from build123d import *

# Parameters (mm, degrees)
SKETCH1_R           = 48.846646741
SKETCH1_R_2         = 45.593095846
BOSS_EXTRUDE1_DEPTH = 10
SKETCH2_W           = 14.682281382
SKETCH2_H           = 11.549997154
SKETCH2_W_2         = 10
SKETCH2_H_2         = 8
BOSS_EXTRUDE2_DEPTH = 15
FILLET1_R           = 4


with BuildPart() as part:
    # Sketch1 → Boss-Extrude1 (new, symmetric)
    with BuildSketch(Plane.XY):
        Circle(SKETCH1_R)
        Circle(SKETCH1_R_2, mode=Mode.SUBTRACT)
    extrude(amount=BOSS_EXTRUDE1_DEPTH, both=True)

    # Sketch2 → Boss-Extrude2 (add)
    with BuildSketch(Plane.XY.offset(10)):
        with Locations((0, 53.899768405)):
            Rectangle(SKETCH2_W, SKETCH2_H)
        with Locations((0, 53.899768405)):
            Rectangle(SKETCH2_W_2, SKETCH2_H_2, mode=Mode.SUBTRACT)
    extrude(amount=-BOSS_EXTRUDE2_DEPTH)

    # Fillet1
    fillet1_edges = [part.edges().sort_by_distance(p)[0] for p in [
        (7.341140691, 59.674766982, 2.5),
        (-7.341140691, 59.674766982, 2.5),
    ]]
    fillet(fillet1_edges, radius=FILLET1_R)


solid = part.part
Can you work these out from the model? Positions are in its coordinate system, mm. A direction names the side the tool comes from. Round coordinates to 2 decimals unless told otherwise and drop trailing zeros. Loops run counter-clockwise (first coordinate to the right, second up) from the corner with the lowest first, then second, coordinate; pieces in that order, holes last. Notation, with made-up numbers: (73, 4) - (84, 4) arc R26 ccw to (84, 38) - close; hole circle Ø1 at (72.5, 36.5). An arc over 180 degrees is marked (long way). Use CSV: the item, a comma, the result in double quotes. Start each with the question number.
1) If we section it at D-D on x = 19.5: Write out the boundary of the cut face in (y, z).
2) If we section it at A-A on z = 7.25: Write out the boundary of the cut face in (x, y), plus the area to 3 significant figures.
3) If we section it at C-C on y = 0: Write out the boundary of the cut face in (x, z), plus the area to 3 significant figures.
4) We'd pull the mould along X, two halves only. Please class faces 5 (the flat face through (0, 57.9, 3)), 6 (the flat face through (0, 46, 10)), 7 (the cylindrical face through (21.04, -40.45, -0.14)), 8 (the cylindrical face through (-6.2, 58.47, 2.39)): released by +X, released by -X, zero draft, split by the parting line, or undercut.
5) For pin 1 Ø4 at (x, z) = (5.5, -2.5) entering from +Y; pin 2 Ø6.5 at (y, z) = (54.5, 5) entering from -X; pin 3 Ø4 at (y, z) = (8, -0.5) entering from -X; pin 4 Ø8 at (y, z) = (4, -0.5) entering from +X, each with a flat end and sliding along its axis, tell me the tip position at first contact or that it passes through.
6) If we section it at B-B on x = 0: Write out the boundary of the cut face in (y, z), plus the area to 3 significant figures.
7) For faces 1 (the flat face through (0, 59.675, 3)), 2 (the flat face through (-7.341, 52, 3)), 3 (the flat face through (-5, 54, 3)), 4 (the flat face through (7.341, 52, 3)), which set-ups out of +Z, -Z, +X, -X, +Y, -Y let a thin tool reach every point of the face, with its end or its side?
8) Please list where these lines run through material, in increasing order: probe 1 along Y at (x, z) = (0, -4); probe 2 along Y at (x, z) = (34.5, -6.5); probe 3 along Y at (x, z) = (24, -0.25). Write a range as [from, to].
Geometry results:
1,outline,"(-44.79, -10) - (-41.21, -10) - (-41.21, 10) - (-44.79, 10) - close; (41.21, -10) - (44.79, -10) - (44.79, 10) - (41.21, 10) - close"
2,outline,"(-7.34, 48.29) arc R48.85 ccw (long way) to (7.34, 48.29) - (7.34, 55.67) arc R4 ccw to (3.34, 59.67) - (-3.34, 59.67) arc R4 ccw to (-7.34, 55.67) - close; hole circle Ø91.19 at (0, 0); hole (-5, 49.9) - (5, 49.9) - (5, 57.9) - (-5, 57.9) - close"
2,area,"1,040 mm2"
3,outline,"(-48.85, -10) - (-45.59, -10) - (-45.59, 10) - (-48.85, 10) - close; (45.59, -10) - (48.85, -10) - (48.85, 10) - (45.59, 10) - close"
3,area,"130 mm2"
4,face 5,"undercut"
4,face 6,"zero draft"
4,face 7,"undercut"
4,face 8,"released by -X"
5,pin 1,"stops at y = 59.67"
5,pin 2,"stops at x = -7.34"
5,pin 3,"stops at x = -48.48"
5,pin 4,"stops at x = 48.85"
6,outline,"(-48.85, -10) - (-45.59, -10) - (-45.59, 10) - (-48.85, 10) - close; (45.59, -10) - (48.85, -10) - (48.85, -5) - (49.9, -5) - (49.9, 10) - (45.59, 10) - close; (57.9, -5) - (59.67, -5) - (59.67, 10) - (57.9, 10) - close"
6,area,"173 mm2"
7,face 1,"+Z, -Z, +X, -X, +Y"
7,face 2,"+Z, -Z, -X, +Y"
7,face 3,"+Z, -Z"
7,face 4,"+Z, -Z, +X, +Y"
8,probe 1,"y = [-48.85, -45.59], [45.59, 49.9], [57.9, 59.67]"
8,probe 2,"y = [-34.58, -29.81], [29.81, 34.58]"
8,probe 3,"y = [-42.54, -38.77], [38.77, 42.54]"
